Can you work these out from the drawing? Everything is in mm from the part's minimum corner. A direction names the side the tool comes from. Coordinates: 2 decimals unless noted, no trailing zeros. Order: outer loops, then holes, each group sorted by start corner. A loop starts at its lowest first (then second) coordinate and runs counter-clockwise, first axis right, second up. Notation, with made-up numbers: (81, 26) -> (90, 26) arc R14 ccw to (90, 51) -> close; hole circle Ø8 at (76, 71). An arc over 180 degrees is marked (long way). Return JSON: item names as keys, results as strings. Group by question number.
1) For pin 1 (1 mm diameter, centred on y = 47, z = 0.5, fed in from -X); pin 2 (1.5 mm diameter, centred on x = 27.5, z = 2, fed in from -Y), each with a flat end and sliding along its axis, tell me the tip position at first contact or that it passes through.
2) Thinking about a two-plate mould opening in X: for the marked faces 1 and 2, which applies, +X half, -X half, draft (parallel to the pull), parting line (faces both ways), or undercut?
3) If we section it at A-A, the plane y = 22.5: Please give me the cut outline in (x, z), then the cut area to 3 significant figures.
4) If I drill on probe 1 along X at (y, z) = (43.5, 4.2); probe 2 along Y at (x, z) = (12.5, 3.25); probe 3 along Y at (x, z) = (39, 3.15), over which ranges is the centre line in solid material (lowest first)? Write a range as from..to.
5) If we section it at C-C, the plane y = 12.5: Please give me the cut outline in (x, z).
6) If we section it at B-B, the plane z = 2.05: Please give me the cut outline in (x, y), then the cut area to 3 significant figures.
7) For the marked faces 3, 4, 5 and 6, which set-ups out of +Z, -Z, +X, -X, +Y, -Y let a thin tool reach every point of the face, with its end or its side?
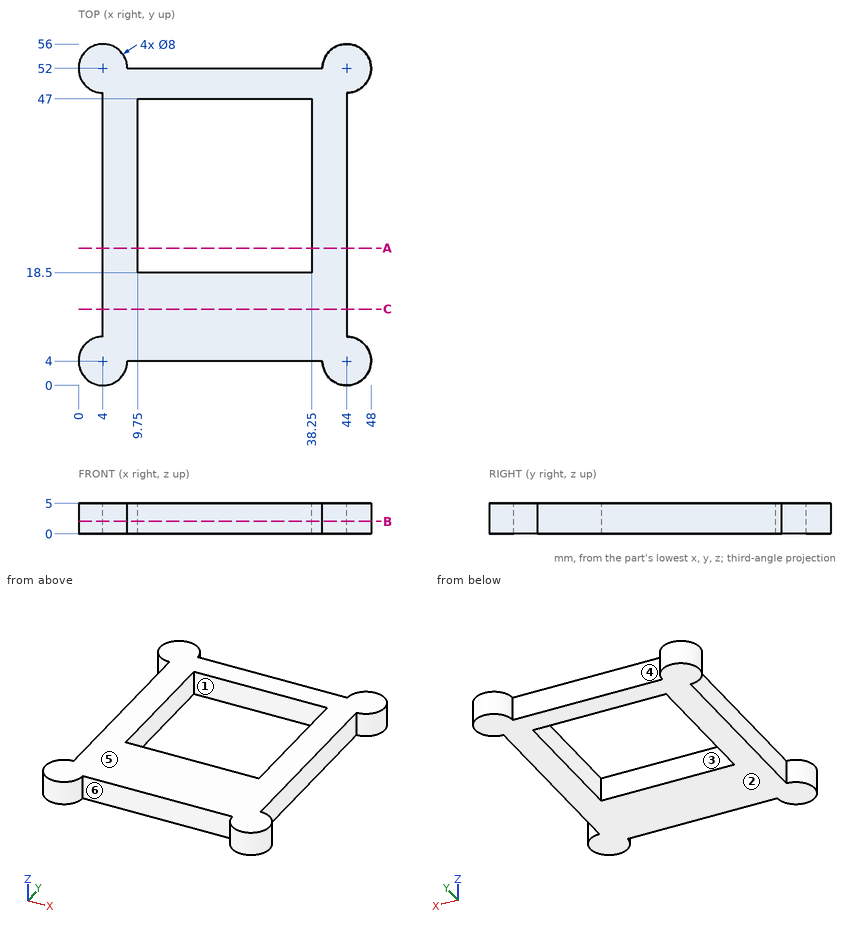
Result sheet:
{
 "1": {"pin 1": "stops at x = 4", "pin 2": "stops at y = 4"},
 "2": {"face 1": "undercut", "face 2": "draft"},
 "3": {"outline": "(4, 0) -> (9.75, 0) -> (9.75, 5) -> (4, 5) -> close; (38.25, 0) -> (44, 0) -> (44, 5) -> (38.25, 5) -> close", "area": "57.5 mm2"},
 "4": {"probe 1": "x = 4..9.75, 38.25..44", "probe 2": "y = 4..18.5, 47..52", "probe 3": "y = 4..52"},
 "5": {"outline": "(4, 0) -> (44, 0) -> (44, 5) -> (4, 5) -> close"},
 "6": {"outline": "(4, 8) arc R4 ccw (long way) to (8, 4) -> (40, 4) arc R4 ccw (long way) to (44, 8) -> (44, 48) arc R4 ccw (long way) to (40, 52) -> (8, 52) arc R4 ccw (long way) to (4, 48) -> close; hole (9.75, 18.5) -> (38.25, 18.5) -> (38.25, 47) -> (9.75, 47) -> close", "area": "1,260 mm2"},
 "7": {"face 3": "+Z, -Z", "face 4": "+Z, -Z, +Y", "face 5": "+Z, +X, -X, +Y, -Y", "face 6": "+Z, -Z, -Y"}
}
